Read the model definition and answer for the solid it produces. Units are mm, in the model's axes. Coordinates: 2 decimals unless noted, no trailing zeros. Loops run counter-clockwise (first coordinate to the right, second up) from the corner with the lowest first, then second, coordinate; pieces in that order, holes last. Notation, with made-up numbers: (-37, 70) -> (19, 70) arc R21 cw to (19, 95) -> close; hole circle Ø5 at (57.5, -21.5). An arc over 180 degrees is marked (long way). Answer as a JSON object with one key per item and string values. Group by question number.
Q1. The part is cut by section D-D on x = 16. Write down the section's boundary in (y, z).
Q2. The part is cut by section C-C on y = 2.5. Write down the section's boundary in (x, z).
Q3. The part is cut by section B-B on z = 15. Write down the section's boundary in (x, y), and give its area (3 significant figures).
Q4. This flat-tipped pin is pushed along its axis until it touches: P1, Ø13, axis at x = 50, z = 60, coming from the +Y side. Where does it stop, or does it pass through?
Q5. The part is cut by section A-A on x = 79. Write down the section's boundary in (y, z), and give its area (3 significant figures).
Q6. Straight lines are drawn through the part: line 1 along Z through (x, y) = (41.5, 0.75); line 2 along Z through (x, y) = (101.5, 2.75); line 3 along X through (y, z) = (2, 21). For each, find the intervals that lie inside material, in ascending order. Write a range as [from, to].
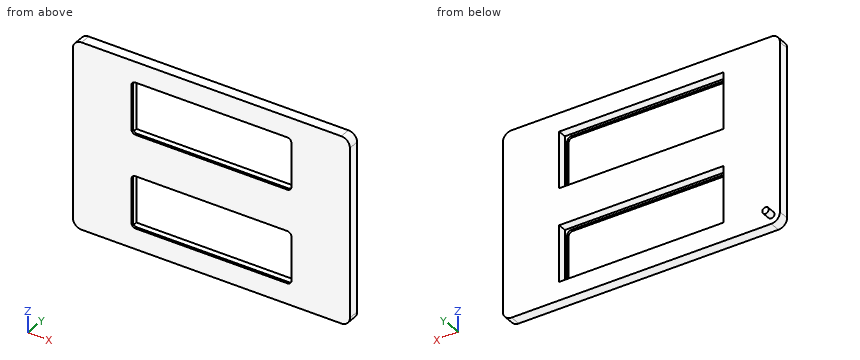
Autodesk Fusion 360 part; units mm, degrees
sketch "Sketch1" plane through (0, 0, 0) normal (0, 1, 0) x (1, 0, 0)
  line L0 (5, -15) -> (56.3866, -15)
  line L1 (56.3866, -15) -> (56.3866, -37.4714)
  line L2 (56.3866, -37.4714) -> (5, -37.4714)
  line L3 (5, -37.4714) -> (5, -15)
sketch "Sketch2" plane through (0, 0, 0) normal (0, 1, 0) x (1, 0, 0)
  line L0 (4, 0) -> (124, 0)
  line L1 (128, -4) -> (128, -82)
  line L2 (124, -86) -> (4, -86)
  line L3 (0, -82) -> (0, -4)
  arc A0 (4, 0) -> (0, -4) centre (4, -4) ccw
  arc A1 (128, -4) -> (124, 0) centre (124, -4) ccw
  arc A2 (0, -82) -> (4, -86) centre (4, -82) ccw
  arc A3 (124, -86) -> (128, -82) centre (124, -82) ccw
  line L4 (64, -86) -> (64, 0) construction
  line L5 (64, -43) -> (64, -21.5) construction
  line L6 (64, -21.5) -> (64, -8.5) construction
  line L7 (64, -8.5) -> (26, -8.5) construction
  line L8 (26, -8.5) -> (102, -8.5)
  line L9 (102, -8.5) -> (102, -34.5)
  line L10 (102, -34.5) -> (26, -34.5)
  line L11 (26, -34.5) -> (26, -8.5)
  line L12 (26, -8.5) -> (27, -8.5) construction
  line L13 (27, -8.5) -> (27, -9.5) construction
  line L14 (29, -9.5) -> (99, -9.5)
  line L15 (101, -11.5) -> (101, -31.5)
  line L16 (99, -33.5) -> (29, -33.5)
  line L17 (27, -31.5) -> (27, -11.5)
  line L18 (64, -64.5) -> (64, -77.5) construction
  line L19 (64, -77.5) -> (26, -77.5) construction
  line L20 (26, -77.5) -> (102, -77.5)
  line L21 (102, -77.5) -> (102, -51.5)
  line L22 (102, -51.5) -> (26, -51.5)
  line L23 (26, -51.5) -> (26, -77.5)
  line L24 (26, -77.5) -> (26, -76.5)
  line L25 (26, -76.5) -> (27, -76.5)
  line L26 (29, -76.5) -> (99, -76.5)
  line L27 (101, -74.5) -> (101, -54.5)
  line L28 (99, -52.5) -> (29, -52.5)
  line L29 (27, -54.5) -> (27, -74.5)
  arc A4 (29, -52.5) -> (27, -54.5) centre (29, -54.5) ccw
  arc A5 (27, -74.5) -> (29, -76.5) centre (29, -74.5) ccw
  arc A6 (101, -54.5) -> (99, -52.5) centre (99, -54.5) ccw
  arc A7 (99, -76.5) -> (101, -74.5) centre (99, -74.5) ccw
  arc A8 (29, -9.5) -> (27, -11.5) centre (29, -11.5) ccw
  arc A9 (27, -31.5) -> (29, -33.5) centre (29, -31.5) ccw
  arc A10 (99, -33.5) -> (101, -31.5) centre (99, -31.5) ccw
  arc A11 (101, -11.5) -> (99, -9.5) centre (99, -11.5) ccw
  circle A12 centre (4, -4) radius 1.5
  point P0 (128, 0)
  point P1 (0, -86)
  point P2 (101, -9.5)
  point P3 (27, -33.5)
  point P4 (101, -76.5)
  point P5 (27, -52.5)
  dimension "d3" = 128
  dimension "d4" = 86
  dimension "d5" = 4
  dimension "d6" = 4
  dimension "d7" = 4
  dimension "d8" = 4
  dimension "d12" = 76
  dimension "d13" = 26
  dimension "d14" = 1
  dimension "d15" = 74
  dimension "d16" = 24
  dimension "d20" = 76
  dimension "d21" = 26
  dimension "d22" = 74
  dimension "d23" = 24
  dimension "d24" = 2
  dimension "d25" = 2
  dimension "d26" = 2
  dimension "d27" = 2
  dimension "d28" = 2
  dimension "d29" = 2
  dimension "d30" = 2
  dimension "d31" = 2
  dimension "d32" = 3
extrude "Extrude2" add sketch "Sketch2" along normal blind 5 contours L0 L1 L2 L3 A0 A1 A2 A3
extrude "Extrude3" add sketch "Sketch2" along normal blind 0.5 contours L8 L9 L10 L11
extrude "Extrude4" add 1 faces at (52.3333, 0.5, 34.1667) along direction (0, 1, 0) blind 0.5
extrude "Extrude5" add sketch "Sketch2" along normal blind 1 contours L20 L21 L22 L23 L24
extrude "Extrude6" add sketch "Sketch2" along normal blind 12 contours A12
extrude "Extrude7" cut 1 faces at (3.584, 12, 3.3234) along direction (0, -1, 0) blind 5
extrude "Extrude8" add 1 faces at (3.584, 7, 3.3234) along direction (0, 1, 0) blind 2
Final values:
{
 "1": {"outline": "(0, 0) -> (5, 0) -> (5, 86) -> (0, 86) -> close"},
 "2": {"outline": "(0, 4) arc R4 ccw to (4, 0) -> (124, 0) arc R4 ccw to (128, 4) -> (128, 82) arc R4 ccw to (124, 86) -> (4, 86) arc R4 ccw to (0, 82) -> close; hole (26, 8.5) -> (102, 8.5) -> (102, 34.5) -> (26, 34.5) -> close; hole (26, 51.5) -> (102, 51.5) -> (102, 77.5) -> (26, 77.5) -> close"},
 "3": {"outline": "(0, 0) -> (27, 0) -> (27, 1) -> (26, 1) -> (26, 5) -> (0, 5) -> close; (101, 0) -> (128, 0) -> (128, 5) -> (102, 5) -> (102, 1) -> (101, 1) -> close", "area": "262 mm2"},
 "4": {"P1": "passes through"},
 "5": {"outline": "(0, 0) -> (5, 0) -> (5, 8.5) -> (1, 8.5) -> (1, 9.5) -> (0, 9.5) -> close; (0, 33.5) -> (1, 33.5) -> (1, 34.5) -> (5, 34.5) -> (5, 51.5) -> (1, 51.5) -> (1, 52.5) -> (0, 52.5) -> close; (0, 76.5) -> (1, 76.5) -> (1, 77.5) -> (5, 77.5) -> (5, 86) -> (0, 86) -> close", "area": "174 mm2"},
 "6": {"line 1": "z = [0, 9.5], [33.5, 52.5], [76.5, 86]", "line 2": "z = [0, 8.5], [34.5, 51.5], [77.5, 86]", "line 3": "x = [0, 26], [102, 128]"}
}
